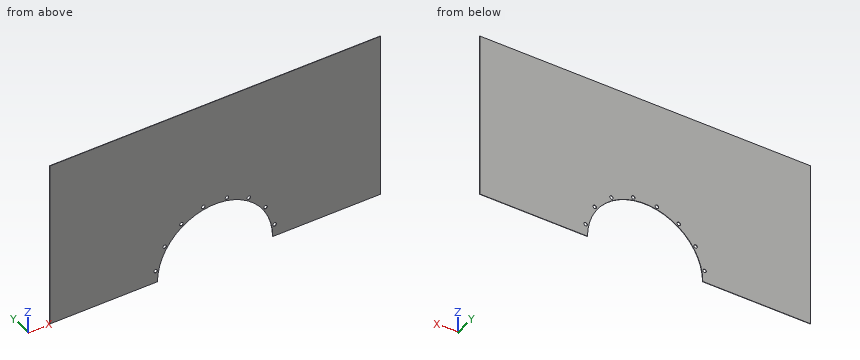
```python
from build123d import *

# Parameters (mm, degrees)
SKETCH2_R           = 6.5
BOSS_EXTRUDE2_DEPTH = 1.5875


with BuildPart() as part:
    # Sketch2 → Boss-Extrude2 (new body)
    with BuildSketch(Plane(origin=(0, 0, 0), x_dir=(1, 0, 0), z_dir=(0, 1, 0))):
        with BuildLine():
            ThreePointArc((-212.625, 0), (0, -212.625), (212.625, 0))
            Line((212.625, 0), (609.6, 0))
            Line((609.6, 0), (609.6, -609.6))
            Line((609.6, -609.6), (-609.6, -609.6))
            Line((-609.6, -609.6), (-609.6, 0))
            Line((-609.6, 0), (-212.625, 0))
        make_face()
        with Locations(Location((-219.20551017, -43.602686971, 0), (0, 0, 270))):
            Circle(SKETCH2_R, mode=Mode.SUBTRACT)
        with Locations(Location((-185.83345835, -124.16994708, 0), (0, 0, 270))):
            Circle(SKETCH2_R, mode=Mode.SUBTRACT)
        with Locations(Location((-124.16994708, -185.83345835, 0), (0, 0, 270))):
            Circle(SKETCH2_R, mode=Mode.SUBTRACT)
        with Locations(Location((-43.602686971, -219.20551017, 0), (0, 0, 270))):
            Circle(SKETCH2_R, mode=Mode.SUBTRACT)
        with Locations(Location((43.602686971, -219.20551017, 0), (0, 0, 270))):
            Circle(SKETCH2_R, mode=Mode.SUBTRACT)
        with Locations(Location((124.16994708, -185.83345835, 0), (0, 0, 270))):
            Circle(SKETCH2_R, mode=Mode.SUBTRACT)
        with Locations(Location((185.83345835, -124.16994708, 0), (0, 0, 270))):
            Circle(SKETCH2_R, mode=Mode.SUBTRACT)
        with Locations(Location((219.20551017, -43.602686971, 0), (0, 0, 270))):
            Circle(SKETCH2_R, mode=Mode.SUBTRACT)
    extrude(amount=BOSS_EXTRUDE2_DEPTH)


solid = part.part
```
Could you check a few things on this model? Use its own coordinates, in mm. Round coordinates to 2 decimals unless told otherwise and drop trailing zeros. Loops run counter-clockwise (first coordinate to the right, second up) from the corner with the lowest first, then second, coordinate; pieces in that order, holes last. Notation, with made-up numbers: M -7,51 L 37,51 A28 ccw 37,89 Z; hole C 86.25,56 d1. An arc over 180 degrees is marked long. Write item = value, one per line.
1. Will this pin go through, and if not, where does the flat tip stop? P1, Ø1.5, axis at x = -333.5, z = 515.5, coming from the -Y side.
Results below:
P1 = 0
2. I want a section at B-B, the plane x = 0. Write out the boundary of the cut face in (y, z) (1 decimal), and give its area (3 significant figures).
Results below:
outline = M 0,212.6 L 1.6,212.6 L 1.6,609.6 L 0,609.6 Z
area = 630 mm²
3. I want a section at A-A, the plane y = 0.7. Count the separate pieces of the cut face and the enclosed holes in it, and give its area (3 significant figures).
Results below:
separate_pieces = 1
enclosed_holes = 8
area = 671,000 mm²
4. I need wall thicknesses on probe 1 along X at (y, z) = (1.2, 47.5); probe 2 along X at (y, z) = (0.7, 46); probe 3 along X at (y, z) = (0.3, 73). Which ranges of each line are inside material? Lowest first, please.
Results below:
probe_1 = -609.6 to -224.41, -214 to -207.25, 207.25 to 214, 224.41 to 609.6
probe_2 = -609.6 to -225.25, -213.16 to -207.59, 207.59 to 213.16, 225.25 to 609.6
probe_3 = -609.6 to -199.7, 199.7 to 609.6
